For this review, take the finished solid that the model builds, in its own axes (mm). Round coordinates to 2 decimals unless told otherwise and drop trailing zeros. Order: outer loops, then holes, each group sorted by start corner. A loop starts at its lowest first (then second) coordinate and runs counter-clockwise, first axis right, second up. Notation, with made-up numbers: (36, 82.25) - (84, 82.25) arc R8 ccw to (84, 90.25) - close; hole circle Ø1 at (40.25, -21.75). An arc over 180 degrees is marked (long way). One line per item, written item: value.
```python
from build123d import *

# Parameters (mm, degrees)
F0_W     = 266.5
F0_H     = 160
F0_R     = 3
F1_DEPTH = 4
F2_R     = 3
F3_DEPTH = 4.001
F4_W     = 25.75
F4_H     = 23
F4_W_2   = 82.5
F4_H_2   = 32
F5_DEPTH = 4.001
F6_W     = 70
F6_H     = 19.5
F7_DEPTH = 4.001


with BuildPart() as f1:
    # F0 (on Top) → F1 (new body)
    with BuildSketch(Plane.XY):
        Rectangle(F0_W, F0_H)
        with Locations((-123, -44.5)):
            Circle(F0_R, mode=Mode.SUBTRACT)
        with Locations((123, -44.5)):
            Circle(F0_R, mode=Mode.SUBTRACT)
        with Locations((-123, 44.5)):
            Circle(F0_R, mode=Mode.SUBTRACT)
        with Locations((123, 44.5)):
            Circle(F0_R, mode=Mode.SUBTRACT)
    extrude(amount=F1_DEPTH)

    # F2 (on face) → F3 (cut, through all)
    with BuildSketch(Plane.XY.offset(4)):
        with Locations((-95, 70)):
            Circle(F2_R)
        with Locations((-95, -70)):
            Circle(F2_R)
        with Locations((95, 70)):
            Circle(F2_R)
        with Locations((95, -70)):
            Circle(F2_R)
    extrude(amount=-F3_DEPTH, mode=Mode.SUBTRACT)

    # F4 (on face) → F5 (cut, through all)
    with BuildSketch(Plane.XY.offset(4)):
        with Locations((-120.375, 68.5)):
            Rectangle(F4_W, F4_H)
        with Locations((-41.25, 68.5)):
            Rectangle(F4_W_2, F4_H)
        with Locations((41.25, 68.5)):
            Rectangle(F4_W_2, F4_H)
        with Locations((-120.375, 16)):
            Rectangle(F4_W, F4_H_2)
        with Locations((-120.375, -16)):
            Rectangle(F4_W, F4_H_2)
        with Locations((120.375, 68.5)):
            Rectangle(F4_W, F4_H)
        with Locations((120.375, 16)):
            Rectangle(F4_W, F4_H_2)
        with Locations((120.375, -16)):
            Rectangle(F4_W, F4_H_2)
        with Locations((-41.25, -68.5)):
            Rectangle(F4_W_2, F4_H)
        with Locations((41.25, -68.5)):
            Rectangle(F4_W_2, F4_H)
        with Locations((-120.375, -68.5)):
            Rectangle(F4_W, F4_H)
        with Locations((120.375, -68.5)):
            Rectangle(F4_W, F4_H)
    extrude(amount=-F5_DEPTH, mode=Mode.SUBTRACT)

    # F6 (on face) → F7 (cut, through all)
    with BuildSketch(Plane.XY.offset(4)):
        with Locations((-47.5, 22.25)):
            Rectangle(F6_W, F6_H)
        with Locations((47.5, 22.25)):
            Rectangle(F6_W, F6_H)
        with Locations((47.5, -22.25)):
            Rectangle(F6_W, F6_H)
        with Locations((-47.5, -22.25)):
            Rectangle(F6_W, F6_H)
    extrude(amount=-F7_DEPTH, mode=Mode.SUBTRACT)


solid = f1.part
```
Item 1: Take a section at B-B (x = 46). Write out the cut boundary in (y, z).
Returned:
outline: (-57, 0) - (-32, 0) - (-32, 4) - (-57, 4) - close; (-12.5, 0) - (12.5, 0) - (12.5, 4) - (-12.5, 4) - close; (32, 0) - (57, 0) - (57, 4) - (32, 4) - close
Item 2: The part is to be moulded in two halves that separate along Y. For faces 1 (the flat face through (-2, 1, 0)), 2 (the cylindrical face through (-97.4, 68.2, 2)), say which applies: +Y half, -Y half, draft (parallel to the pull), parting line (faces both ways), or undercut.
Returned:
face 1: draft
face 2: undercut
Item 3: Take a section at A-A (y = 70). Write out the cut boundary in (x, z).
Returned:
outline: (-107.5, 0) - (-98, 0) - (-98, 4) - (-107.5, 4) - close; (-92, 0) - (-82.5, 0) - (-82.5, 4) - (-92, 4) - close; (82.5, 0) - (92, 0) - (92, 4) - (82.5, 4) - close; (98, 0) - (107.5, 0) - (107.5, 4) - (98, 4) - close
Item 4: Wall thickness on line 1 (X direction, y = 18.5, z = 3.6); line 2 (Y direction, x = -95, z = 1.5); line 3 (Y direction, x = 23.5, z = 1.4): over which ranges is each line inside the solid? List them lowest first.
Returned:
line 1: -107.5 to -82.5, -12.5 to 12.5, 82.5 to 107.5
line 2: -80 to -73, -67 to 67, 73 to 80
line 3: -57 to -32, -12.5 to 12.5, 32 to 57
Item 5: For P1, Ø2, axis at x = -41, z = 2, coming from the -Y side; P2, Ø2, axis at x = 119.5, z = 2.5, coming from the +Y side; P3, Ø2, axis at y = -23.5, z = 2, coming from the +X side, all flat-tipped, find the tip position at first contact; note any pin that passes through.
Returned:
P1: y = -57
P2: y = 57
P3: x = 107.5
Item 6: Take a section at C-C (y = -44.5). Write out the cut boundary in (x, z), plus the area to 3 significant figures.
Returned:
outline: (-133.25, 0) - (-126, 0) - (-126, 4) - (-133.25, 4) - close; (-120, 0) - (120, 0) - (120, 4) - (-120, 4) - close; (126, 0) - (133.25, 0) - (133.25, 4) - (126, 4) - close
area: 1,020 mm^2
Item 7: Take a section at D-D (x = 123). Write out the cut boundary in (y, z).
Returned:
outline: (-57, 0) - (-47.5, 0) - (-47.5, 4) - (-57, 4) - close; (-41.5, 0) - (-32, 0) - (-32, 4) - (-41.5, 4) - close; (32, 0) - (41.5, 0) - (41.5, 4) - (32, 4) - close; (47.5, 0) - (57, 0) - (57, 4) - (47.5, 4) - close
